The listing builds one solid part. Answer for the finished solid, in the listing's coordinates (mm). A direction names the side the tool comes from. Give positions to 0.01 mm unless a question says otherwise; leave off trailing zeros. Write each loop counter-clockwise with the first axis right and the second up, starting at its lowest first coordinate (ties: lowest second). Pieces come first, ordered by that corner, then holes. Notation, with made-up numbers: (34.25, 81.25) - (43.25, 81.25) arc R29 ccw to (43.25, 106.25) - close; hole circle Ø7 at (8.25, 36.5). An arc over 180 degrees is marked (long way). Write each question's results on one line, items separated by ' | '. Start each with the question number.
Q1. Find the intervals of material crossed by probe 1 along X at (y, z) = (-15.5, 12.5); probe 2 along X at (y, z) = (-3.5, 32.5); probe 3 along Y at (x, z) = (64.5, 12.5), in increasing order.
Q2. Section D-D (x = 87.5) is taken. Determine the outline of the cut face in (y, z), plus the area to 3 significant figures.
Q3. Flat-ended cylindrical pins translate along their axes: pin 1 Ø4.5 at (x, y) = (-190.11, -14.94) entering from -Z; pin 2 Ø3 at (y, z) = (-47.5, 51.5) entering from +X; pin 3 Ø1.6 at (y, z) = (33.5, 32.5) entering from +X; pin 4 Ø10 at (y, z) = (-11, 64.5) entering from +X. Find the tip coordinate at first contact, or state that the pin passes through.
Q4. For faces 4 (the face through (150, 0, 10)), 5 (the face through (15, -35, 35)), 6 (the face through (150, 0, 60)), 7 (the face through (-199, 0, 20)), determine the directions among +Z, -Z, +X, -X, +Y, -Y from which every point of the face is accessible in a straight line to the end or side of a thin tool.
Q5. Section A-A (z = 35) is taken. Determine the outline of the cut face in (x, y).
Q6. Section C-C (z = 58) is taken. Determine the outline of the cut face in (x, y), plus the area to 3 significant figures.
Q7. For a pull along Y with two mould halves and no side action, classify faces 1 (the face through (15, 35, 35)), 2 (the face through (-52, 1, 0)), 3 (the face through (-166.4, -13.4, 55.2)) as pulls with the +Y half, pulls with the -Y half, needs draft (parallel to the pull), parting line crosses it, or undercut.
Q8. Section B-B (z = 12) is taken. Determine the outline of the cut face in (x, y).
```python
from build123d import *

# Parameters (mm, degrees)
SKETCH_1_W          = 300
SKETCH_1_H          = 70
EXTRUDE_1_DEPTH     = 70
SKETCH_2_R          = 60
EXTRUDE_2_DEPTH     = 70
SKETCH_3_W          = 35
SKETCH_3_H          = 30
EXTRUDE_3_DEPTH     = 70
SKETCH_5_R          = 40
EXTRUDE_5_DEPTH     = 30
SKETCH_6_R          = 15
CUT_EXTRUDE_1_DEPTH = 271.265181117
SKETCH_7_R          = 2
CUT_EXTRUDE_2_DEPTH = 275.669379662
SKETCH_8_R          = 25
CUT_EXTRUDE_3_DEPTH = 50
SKETCH_9_R          = 35
CUT_EXTRUDE_4_DEPTH = 30


with BuildPart() as part:
    # 草图1 → 凸台-拉伸1 (new body)
    with BuildSketch(Plane.XY):
        Rectangle(SKETCH_1_W, SKETCH_1_H)
    extrude(amount=EXTRUDE_1_DEPTH)

    # 草图2 → 凸台-拉伸2 (add)
    with BuildSketch(Plane(origin=(0, 0, 0), x_dir=(-1, 0, 0), z_dir=(0, 0, -1))):
        with Locations((198.733971724, 0)):
            Circle(SKETCH_2_R)
    extrude(amount=-EXTRUDE_2_DEPTH)

    # 草图3 → 凸台-拉伸3 (add)
    with BuildSketch(Plane(origin=(0, 35, 0), x_dir=(1, 0, 0), z_dir=(0, 1, 0))):
        with Locations((167.5, -35)):
            Rectangle(SKETCH_3_W, SKETCH_3_H)
    extrude(amount=-EXTRUDE_3_DEPTH)

    # 草图5 → 凸台-拉伸5 (add)
    with BuildSketch(Plane.XY.offset(50)):
        with Locations((207.605309111, 0)):
            Circle(SKETCH_5_R)
    extrude(amount=-EXTRUDE_5_DEPTH)

    # 草图6 → 切除-拉伸1 (cut, through all)
    with BuildSketch(Plane(origin=(0, 0, 20), x_dir=(-1, 0, 0), z_dir=(0, 0, -1))):
        with Locations((-207.605309111, 0)):
            Circle(SKETCH_6_R)
    extrude(amount=-CUT_EXTRUDE_1_DEPTH, mode=Mode.SUBTRACT)

    # 草图7 → 切除-拉伸2 (cut, through all)
    with BuildSketch(Plane(origin=(0, 0, 0), x_dir=(-1, 0, 0), z_dir=(0, 0, -1))):
        with Locations((215.983971724, 0)):
            Circle(SKETCH_7_R)
        with Locations((207.358971724, -14.938938215)):
            Circle(SKETCH_7_R)
        with Locations((190.108971724, -14.938938215)):
            Circle(SKETCH_7_R)
        with Locations((181.483971724, 0)):
            Circle(SKETCH_7_R)
        with Locations((190.108971724, 14.938938215)):
            Circle(SKETCH_7_R)
        with Locations((207.358971724, 14.938938215)):
            Circle(SKETCH_7_R)
    extrude(amount=-CUT_EXTRUDE_2_DEPTH, mode=Mode.SUBTRACT)

    # 草图8 → 切除-拉伸3 (cut)
    with BuildSketch(Plane.XY.offset(70)):
        with Locations((-198.733971724, 0)):
            Circle(SKETCH_8_R)
    extrude(amount=-CUT_EXTRUDE_3_DEPTH, mode=Mode.SUBTRACT)

    # 草图9 → 切除-拉伸4 (cut)
    with BuildSketch(Plane.XY.offset(70)):
        with Locations((-198.733971724, 0)):
            Circle(SKETCH_9_R)
    extrude(amount=-CUT_EXTRUDE_4_DEPTH, mode=Mode.SUBTRACT)


solid = part.part
```
Answers below:
1) probe 1: x = -256.7 to -209.28, -205.44 to -192.03, -188.19 to 150 | probe 2: x = -258.63 to -223.49, -173.98 to 193.02, 222.19 to 247.45 | probe 3: y = -35 to 35
2) outline: (-35, 0) - (35, 0) - (35, 70) - (-35, 70) - close | area: 4,900 mm2
3) pin 1: stops at z = 0 | pin 2: stops at x = -160.21 | pin 3: stops at x = 230.64 | pin 4: stops at x = 150
4) face 4: -Z, +X, +Y, -Y | face 5: +Z, -Z, -Y | face 6: +Z, +X, +Y, -Y | face 7: +Z
5) outline: (-150, -35) - (185, -35) - (185, -33) arc R40 ccw (long way) to (185, 33) - (185, 35) - (-150, 35) arc R60 ccw (long way) to start; hole circle Ø50 at (-198.73, 0); hole circle Ø30 at (207.61, 0)
6) outline: (-150, -35) - (150, -35) - (150, 35) - (-150, 35) arc R60 ccw (long way) to start; hole circle Ø70 at (-198.73, 0) | area: 27,900 mm2
7) face 1: pulls with the +Y half | face 2: needs draft | face 3: undercut
8) outline: (-150, -35) - (150, -35) - (150, 35) - (-150, 35) arc R60 ccw (long way) to start; hole circle Ø4 at (-215.98, 0); hole circle Ø4 at (-207.36, -14.94); hole circle Ø4 at (-207.36, 14.94); hole circle Ø4 at (-190.11, -14.94); hole circle Ø4 at (-190.11, 14.94); hole circle Ø4 at (-181.48, 0)
